The model under review builds one solid part; all positions refer to its coordinate system, in mm. A direction names the side the tool comes from. Round coordinates to 2 decimals unless told otherwise and drop trailing zeros. Write each loop counter-clockwise with the first axis right and the second up, starting at its lowest first coordinate (ties: lowest second). Pieces come first, ordered by that corner, then holes. Notation, with made-up numbers: (-18.5, 68) -> (-11.5, 68) arc R20 cw to (-11.5, 104) -> close; hole circle Ø3 at (53, -35.5). An arc over 180 degrees is marked (long way). Answer in a Markdown table with one row per item. Add a question column.
```python
from build123d import *

# Parameters (mm, degrees)
SKETCH1_W               = 144.4879
SKETCH1_H               = 47.625
SKETCH1_R               = 14.3129
BOSS_EXTRUDE1_DEPTH     = 6.35
FILLET1_R               = 12.7
F_10_32_TAPPED_HOLE1_D  = 4.0386
F_10_CLEARANCE_HOLE1_D  = 5.1054
CUT_EXTRUDE2_DEPTH      = 147.5745916
CUT_EXTRUDE2_DEPTH_BACK = 147.5745916
DELETEFACE1_OUTLINE_W   = 6.35
DELETEFACE1_OUTLINE_H   = 31.75
DELETEFACE1_DEPTH       = 5
FILLET3_R               = 12.7
CUT_EXTRUDE1_DEPTH      = 147.5745916
CUT_EXTRUDE3_DEPTH      = 147.5745916
CUT_EXTRUDE3_DEPTH_BACK = 147.5745916
FILLET2_R               = 2.54
DELETEFACE2_DEPTH       = 6.35
FILLET4_R               = 25.4


with BuildPart() as part:
    # Sketch1 → Boss-Extrude1 (new body)
    with BuildSketch(Plane(origin=(0, 0, 0), x_dir=(0, 0, -1), z_dir=(1, 0, 0))):
        with Locations((-72.24395, 0)):
            Rectangle(SKETCH1_W, SKETCH1_H)
        with Locations((-120.65, 0)):
            Circle(SKETCH1_R, mode=Mode.SUBTRACT)
    extrude(amount=BOSS_EXTRUDE1_DEPTH)

    # Fillet1
    fillet1_edges = [part.edges().sort_by_distance(p)[0] for p in [
        (3.175, -23.8125, 144.4879),
        (3.175, 23.8125, 144.4879),
        (3.175, 23.8125, 0),
        (3.175, -23.8125, 0),
    ]]
    fillet(fillet1_edges, radius=FILLET1_R)

    # #10-32 Tapped Hole1 (through all)
    with Locations(Plane.ZY):
        with Locations((103.1875, 17.4625), (138.1125, 17.4625), (138.1125, -17.4625), (103.1875, -17.4625)):
            Hole(F_10_32_TAPPED_HOLE1_D / 2)

    # #10 Clearance Hole1 (through all)
    with Locations(Plane(origin=(6.35, 0, 0), x_dir=(0, 0, -1), z_dir=(1, 0, 0))):
        with Locations((-12.7, 14.2875), (-38.1, 14.2875), (-38.1, -11.1125), (-12.7, -11.1125)):
            Hole(F_10_CLEARANCE_HOLE1_D / 2)

    # Sketch9 → Cut-Extrude2 (cut, two sides: drawn at the far end of the back side and taken through both)
    with BuildSketch(Plane(origin=(6.35, 0, 0), x_dir=(0, 0, -1), z_dir=(1, 0, 0)).offset(-CUT_EXTRUDE2_DEPTH_BACK)):
        with BuildLine():
            Line((312.341235999, -20.6375), (0, -20.6375))
            Line((0, -20.6375), (-89.737984171, -20.6375))
            ThreePointArc((-89.737984171, -20.6375), (-93.626549138, -21.4674044), (-96.8375, -23.8125))
            Line((-96.8375, -23.8125), (-305.064990666, -256.617911957))
            Line((-305.064990666, -256.617911957), (-82.038945456, -840.131042898))
            Line((-82.038945456, -840.131042898), (535.36728121, -604.150630941))
            Line((535.36728121, -604.150630941), (312.341235999, -20.6375))
        make_face()
    extrude(amount=CUT_EXTRUDE2_DEPTH + CUT_EXTRUDE2_DEPTH_BACK, mode=Mode.SUBTRACT)

    # DeleteFace1: read off the stored shape, not the designer's step
    # DeleteFace1 outline → DeleteFace1 (add)
    with BuildSketch(Plane.XY):
        with Locations((3.175, -4.7625)):
            Rectangle(DELETEFACE1_OUTLINE_W, DELETEFACE1_OUTLINE_H)
    extrude(amount=DELETEFACE1_DEPTH)

    # Fillet3
    fillet3_edges = [part.edges().sort_by_distance(p)[0] for p in [
        (3.175, -23.8125, 96.8375),
        (3.175, -20.6375, 0),
    ]]
    fillet(fillet3_edges, radius=FILLET3_R)

    # Sketch8 → Cut-Extrude1 (cut, through all)
    with BuildSketch(Plane(origin=(6.35, 0, 0), x_dir=(0, 0, -1), z_dir=(1, 0, 0))):
        with BuildLine():
            ThreePointArc((-34.03708705, -13.597282609), (-33.343854424, -11.358438021), (-33.802467985, -9.060032015))
            Line((-33.802467985, -9.060032015), (-25.4, -0.65756403))
            Line((-25.4, -0.65756403), (-16.997532015, -9.060032015))
            ThreePointArc((-16.997532015, -9.060032015), (-17.456145576, -11.358438021), (-16.76291295, -13.597282609))
            ThreePointArc((-16.76291295, -13.597282609), (-16.714212781, -16.164584503), (-18.929799856, -17.4625))
            Line((-18.929799856, -17.4625), (-31.870200144, -17.4625))
            ThreePointArc((-31.870200144, -17.4625), (-34.085787219, -16.164584503), (-34.03708705, -13.597282609))
        make_face()
        with BuildLine():
            ThreePointArc((-8.144565217, 12.898464294), (-10.781394154, 9.928560008), (-14.752467985, 9.989967985))
            Line((-14.752467985, 9.989967985), (-23.15493597, 1.5875))
            Line((-23.15493597, 1.5875), (-14.752467985, -6.814967985))
            ThreePointArc((-14.752467985, -6.814967985), (-10.781394154, -6.753560008), (-8.144565217, -9.723464294))
            ThreePointArc((-8.144565217, -9.723464294), (-5.340497431, -11.494884855), (-3.175, -8.982645251))
            Line((-3.175, -8.982645251), (-3.175, 12.157645251))
            ThreePointArc((-3.175, 12.157645251), (-5.340497431, 14.669884855), (-8.144565217, 12.898464294))
        make_face()
        with BuildLine():
            Line((-32.854039054, 20.6375), (-17.945960946, 20.6375))
            ThreePointArc((-17.945960946, 20.6375), (-16.10842501, 19.472959326), (-16.37707543, 17.314135514))
            ThreePointArc((-16.37707543, 17.314135514), (-17.427358043, 14.864987824), (-16.997532015, 12.235032015))
            Line((-16.997532015, 12.235032015), (-25.4, 3.83256403))
            Line((-25.4, 3.83256403), (-33.802467985, 12.235032015))
            ThreePointArc((-33.802467985, 12.235032015), (-33.372641957, 14.864987824), (-34.42292457, 17.314135514))
            ThreePointArc((-34.42292457, 17.314135514), (-34.69157499, 19.472959326), (-32.854039054, 20.6375))
        make_face()
        with BuildLine():
            ThreePointArc((-47.625, 12.157645251), (-45.459502569, 14.669884855), (-42.655434783, 12.898464294))
            ThreePointArc((-42.655434783, 12.898464294), (-40.018605846, 9.928560008), (-36.047532015, 9.989967985))
            Line((-36.047532015, 9.989967985), (-27.64506403, 1.5875))
            Line((-27.64506403, 1.5875), (-36.047532015, -6.814967985))
            ThreePointArc((-36.047532015, -6.814967985), (-40.018605846, -6.753560008), (-42.655434783, -9.723464294))
            ThreePointArc((-42.655434783, -9.723464294), (-45.459502569, -11.494884855), (-47.625, -8.982645251))
            Line((-47.625, -8.982645251), (-47.625, 12.157645251))
        make_face()
        with BuildLine():
            ThreePointArc((-88.423043936, 13.28129417), (-89.618027137, 16.835627136), (-86.591838031, 19.05))
            Line((-86.591838031, 19.05), (-53.975, 19.05))
            ThreePointArc((-53.975, 19.05), (-51.72993597, 18.12006403), (-50.8, 15.875))
            Line((-50.8, 15.875), (-50.8, -7.153111257))
            ThreePointArc((-50.8, -7.153111257), (-52.514427124, -9.972216057), (-55.806205905, -9.746817086))
            Line((-55.806205905, -9.746817086), (-88.423043936, 13.28129417))
        make_face()
        with BuildLine():
            ThreePointArc((-60.801956064, -10.10629417), (-59.606972863, -13.660627136), (-62.633161969, -15.875))
            Line((-62.633161969, -15.875), (-95.25, -15.875))
            ThreePointArc((-95.25, -15.875), (-97.49506403, -14.94506403), (-98.425, -12.7))
            Line((-98.425, -12.7), (-98.425, 10.328111257))
            ThreePointArc((-98.425, 10.328111257), (-96.710572876, 13.147216057), (-93.418794095, 12.921817086))
            Line((-93.418794095, 12.921817086), (-60.801956064, -10.10629417))
        make_face()
    extrude(amount=-CUT_EXTRUDE1_DEPTH, mode=Mode.SUBTRACT)

    # Sketch10 → Cut-Extrude3 (cut, two sides: drawn at the far end of the back side and taken through both)
    with BuildSketch(Plane(origin=(6.35, 0, 0), x_dir=(0, 0, -1), z_dir=(1, 0, 0)).offset(-CUT_EXTRUDE3_DEPTH_BACK)):
        with BuildLine():
            Line((132.08732827, -20.6375), (-89.737984171, -20.6375))
            Line((-89.737984171, -20.6375), (-93.767675351, -20.6375))
            Line((-93.767675351, -20.6375), (-102.360500554, -22.152646924))
            ThreePointArc((-102.360500554, -22.152646924), (-104.611498636, -22.007126952), (-106.543048055, -20.842101086))
            ThreePointArc((-106.543048055, -20.842101086), (-110.805342188, -18.396467904), (-115.719429444, -18.400868838))
            ThreePointArc((-115.719429444, -18.400868838), (-120.65, -19.05), (-125.580570556, -18.400868838))
            ThreePointArc((-125.580570556, -18.400868838), (-130.494657812, -18.396467904), (-134.756951945, -20.842101086))
            ThreePointArc((-134.756951945, -20.842101086), (-141.480096045, -20.830096045), (-141.492101086, -14.106951945))
            ThreePointArc((-141.492101086, -14.106951945), (-139.046467904, -9.844657812), (-139.050868838, -4.930570556))
            ThreePointArc((-139.050868838, -4.930570556), (-139.7, 0), (-139.050868838, 4.930570556))
            ThreePointArc((-139.050868838, 4.930570556), (-139.046467904, 9.844657812), (-141.492101086, 14.106951945))
            ThreePointArc((-141.492101086, 14.106951945), (-141.480096045, 20.830096045), (-134.756951945, 20.842101086))
            ThreePointArc((-134.756951945, 20.842101086), (-130.494657812, 18.396467904), (-125.580570556, 18.400868838))
            ThreePointArc((-125.580570556, 18.400868838), (-120.65, 19.05), (-115.719429444, 18.400868838))
            ThreePointArc((-115.719429444, 18.400868838), (-110.805342188, 18.396467904), (-106.543048055, 20.842101086))
            ThreePointArc((-106.543048055, 20.842101086), (-105.379031086, 21.690809089), (-104.014499446, 22.152646924))
            Line((-104.014499446, 22.152646924), (-94.601004871, 23.8125))
            Line((-94.601004871, 23.8125), (123.854282635, 62.332061266))
            Line((123.854282635, 62.332061266), (-317.628130355, 18.523888755))
            Line((-317.628130355, 18.523888755), (-309.39508472, -64.445672511))
            Line((-309.39508472, -64.445672511), (132.08732827, -20.6375))
        make_face()
    extrude(amount=CUT_EXTRUDE3_DEPTH + CUT_EXTRUDE3_DEPTH_BACK, mode=Mode.SUBTRACT)

    # Fillet2
    fillet2_edges = [part.edges().sort_by_distance(p)[0] for p in [
        (3.175, 9.989967985, 36.047532015),
        (3.175, 1.5875, 27.64506403),
        (3.175, -6.814967985, 36.047532015),
        (3.175, -6.814967985, 14.752467985),
        (3.175, 1.5875, 23.15493597),
        (3.175, 9.989967985, 14.752467985),
        (3.175, 12.235032015, 16.997532015),
        (3.175, 3.83256403, 25.4),
        (3.175, 12.235032015, 33.802467985),
        (3.175, -9.060032015, 33.802467985),
        (3.175, -0.65756403, 25.4),
        (3.175, -9.060032015, 16.997532015),
    ]]
    fillet(fillet2_edges, radius=FILLET2_R)

    # DeleteFace2: read off the stored shape, not the designer's step
    # DeleteFace2 outline → DeleteFace2 (add)
    with BuildSketch(Plane.YZ):
        with BuildLine():
            ThreePointArc((22.221939477, 137.941789381), (20.836837959, 141.473340607), (17.310866585, 142.872585457))
            ThreePointArc((17.310866585, 142.872585457), (20.110734558, 140.750141619), (22.221939477, 137.941789381))
        make_face()
        with BuildLine():
            ThreePointArc((-17.310866585, 142.872585457), (-20.836837959, 141.473340607), (-22.221939477, 137.941789381))
            ThreePointArc((-22.221939477, 137.941789381), (-20.110734558, 140.750141619), (-17.310866585, 142.872585457))
        make_face()
    extrude(amount=DELETEFACE2_DEPTH)

    # Fillet4
    fillet4_edges = [part.edges().sort_by_distance(p)[0] for p in [
        (3.175, 23.8125, 94.601004871),
        (3.175, -20.6375, 93.767675351),
    ]]
    fillet(fillet4_edges, radius=FILLET4_R)


solid = part.part
```
1. Add section C-C on z = 82. State how many separate pieces and enclosed holes the cut face has, plus the area to 3 significant figures.
2. Add section B-B on y = 7. Write out the cut boundary in (x, z) (3 decimals).
3. Insertion check: pin 1 Ø1 at (x, y) = (3, 10) entering from +Z; pin 2 Ø6.5 at (y, z) = (-11.11, 38.1) entering from +X; pin 3 Ø4.5 at (y, z) = (14.29, 12.7) entering from +X; pin 4 Ø3 at (x, y) = (3.5, 17.5) entering from -Z. Each pin has a flat end and moves straight along its axis. Give the tip position at first contact, or say it passes through.
4. For L1, parallel to Z at x = 5.75, y = -15; L2, parallel to Y at x = 1, z = 121; L3, parallel to Y at x = 2.25, z = 10.5, list the stretches that pass through material, from the lowest coordinate up.
5. Tool access review of faces 1 (the flat face through (6.35, 0, 72)), 2 (the flat face through (3, -20.638, 52)), 3 (the cylindrical face through (3.13, -9, 17.46)): name each direction out of +Z, -Z, +X, -X, +Y, -Y from which nothing blocks a thin tool from reaching the whole face with its end or side.
6. Add section A-A on z = 129. Write out the cut boundary in (x, y), plus the area to 3 significant figures.
7. Mouldability with a two-part tool opening along Y and no side actions: class faces 4 (the cylindrical face through (3.22, -17.37, 140.13)), 5 (the cylindrical face through (3.22, -20.73, 93.73)), 6 (the cylindrical face through (3.13, 21.68, 105.4)), 7 (the flat face through (0, 0, 72)) as pulls with the +Y half, pulls with the -Y half, needs draft (parallel to the pull), parting line crosses it, or undercut.
Filled in:
| question | item | result |
|---|---|---|
| 1 | separate pieces | 3 |
| 1 | enclosed holes | 0 |
| 1 | area | 85.2 mm² |
| 2 | outline | (0, 0) -> (6.35, 0) -> (6.35, 3.175) -> (0, 3.175) -> close; (0, 17.742) -> (6.35, 17.742) -> (6.35, 22.233) -> (0, 22.233) -> close; (0, 28.567) -> (6.35, 28.567) -> (6.35, 33.058) -> (0, 33.058) -> close; (0, 47.625) -> (6.35, 47.625) -> (6.35, 50.8) -> (0, 50.8) -> close; (0, 79.526) -> (6.35, 79.526) -> (6.35, 85.031) -> (0, 85.031) -> close; (0, 98.425) -> (6.35, 98.425) -> (6.35, 108.166) -> (0, 108.166) -> close; (0, 133.134) -> (6.35, 133.134) -> (6.35, 138.735) -> (0, 138.735) -> close |
| 3 | pin 1 | z = 139.25 |
| 3 | pin 2 | x = 6.35 |
| 3 | pin 3 | through |
| 3 | pin 4 | z = 0.98 |
| 4 | L1 | 2.14 to 16.39, 34.41 to 60.44, 97.44 to 142.19 |
| 4 | L2 | -19.05 to -14.31, 14.31 to 19.05 |
| 4 | L3 | -20.45 to -12.41, -9.82 to -6.89, 10.06 to 12.99, 15.58 to 23.62 |
| 5 | face 1 | +Z, -Z, +X, +Y, -Y |
| 5 | face 2 | -Z, +X, -X, -Y |
| 5 | face 3 | +X, -X |
| 6 | outline | (0, -18.12) -> (6.35, -18.12) -> (6.35, -11.62) -> (0, -11.62) -> close; (0, 11.62) -> (6.35, 11.62) -> (6.35, 18.12) -> (0, 18.12) -> close |
| 6 | area | 82.5 mm² |
| 7 | face 4 | undercut |
| 7 | face 5 | pulls with the -Y half |
| 7 | face 6 | pulls with the +Y half |
| 7 | face 7 | needs draft |
